```python
from build123d import *

# Parameters (mm, degrees)
SKETCH_1_W          = 160
SKETCH_1_H          = 25
EXTRUDE_1_DEPTH     = 4
SKETCH_3_R          = 1.45
CUT_EXTRUDE_1_DEPTH = 4
SKETCH_5_W          = 102
SKETCH_5_H          = 10
EXTRUDE_2_DEPTH     = 8
SKETCH_6_W          = 29
SKETCH_6_H          = 10
CUT_EXTRUDE_2_DEPTH = 6
CHAMFER_1_SIZE      = 10
CUT_EXTRUDE_3_DEPTH = 10
CUT_EXTRUDE_4_DEPTH = 142
SKETCH_10_W         = 122
SKETCH_10_H         = 12
CUT_EXTRUDE_5_DEPTH = 142
CHAMFER_2_SIZE      = 12
SKETCH_11_W         = 15
SKETCH_11_H         = 4
CUT_EXTRUDE_6_DEPTH = 1
SKETCH_12_W         = 15
SKETCH_12_H         = 4
CUT_EXTRUDE_7_DEPTH = 1


with BuildPart() as part:
    # 草图1 → 凸台-拉伸1 (new body)
    with BuildSketch(Plane(origin=(0, 0, 0), x_dir=(1, 0, 0), z_dir=(0, 1, 0))):
        Rectangle(SKETCH_1_W, SKETCH_1_H)
    extrude(amount=EXTRUDE_1_DEPTH)

    # 草图3 → 切除-拉伸1 (cut)
    with BuildSketch(Plane(origin=(0, 4, 0), x_dir=(1, 0, 0), z_dir=(0, 1, 0))):
        with Locations(Location((-75, 7.5, 0), (0, 0, 270))):
            Circle(SKETCH_3_R)
        with Locations(Location((75, 7.5, 0), (0, 0, 270))):
            Circle(SKETCH_3_R)
    extrude(amount=-CUT_EXTRUDE_1_DEPTH, mode=Mode.SUBTRACT)

    # 草图5 → 凸台-拉伸2 (add)
    with BuildSketch(Plane(origin=(0, 4, 0), x_dir=(1, 0, 0), z_dir=(0, 1, 0))):
        with Locations((0, -7.5)):
            Rectangle(SKETCH_5_W, SKETCH_5_H)
    extrude(amount=EXTRUDE_2_DEPTH)

    # 草图6 → 切除-拉伸2 (cut)
    with BuildSketch(Plane(origin=(0, 4, 0), x_dir=(1, 0, 0), z_dir=(0, 1, 0))):
        with Locations((-65.5, -7.5)):
            Rectangle(SKETCH_6_W, SKETCH_6_H)
        with Locations((65.5, -7.5)):
            Rectangle(SKETCH_6_W, SKETCH_6_H)
    extrude(amount=-CUT_EXTRUDE_2_DEPTH, mode=Mode.SUBTRACT)

    # 倒角1
    chamfer_1_edges = [part.edges().sort_by_distance(p)[0] for p in [
        (51, 2, 2.5),
        (-51, 2, 2.5),
    ]]
    chamfer(chamfer_1_edges, length=CHAMFER_1_SIZE - 0.0001)  # a hair under: the kernel refuses the full size

    # 草图7 → 切除-拉伸3 (cut)
    with BuildSketch(Plane(origin=(0, 12, 0), x_dir=(1, 0, 0), z_dir=(0, 1, 0))):
        Polygon((-39.8, -9.3), (-27.4, -9.3), (-27.4, -10.5), (-29.4, -10.5), (-29.4, -12.5), (-37.8, -12.5), (-37.8, -10.5), (-39.8, -10.5), align=None)
        Polygon((-17.4, -9.3), (-5, -9.3), (-5, -10.5), (-7, -10.5), (-7, -12.5), (-15.4, -12.5), (-15.4, -10.5), (-17.4, -10.5), align=None)
        Polygon((5, -9.3), (17.4, -9.3), (17.4, -10.5), (15.4, -10.5), (15.4, -12.5), (7, -12.5), (7, -10.5), (5, -10.5), align=None)
        Polygon((27.4, -9.3), (39.8, -9.3), (39.8, -10.5), (37.8, -10.5), (37.8, -12.5), (29.4, -12.5), (29.4, -10.5), (27.4, -10.5), align=None)
    extrude(amount=-CUT_EXTRUDE_3_DEPTH, mode=Mode.SUBTRACT)

    # 草图9 → 切除-拉伸4 (cut)
    with BuildSketch(Plane.ZY.offset(51)):
        Polygon((7.5, 12), (2.5, 4), (2.5, 12), align=None)
    extrude(amount=-CUT_EXTRUDE_4_DEPTH, mode=Mode.SUBTRACT)

    # 草图10 → 切除-拉伸5 (cut)
    with BuildSketch(Plane(origin=(0, 4, 0), x_dir=(1, 0, 0), z_dir=(0, 1, 0))):
        with Locations((0, 6.5)):
            Rectangle(SKETCH_10_W, SKETCH_10_H)
    extrude(amount=-CUT_EXTRUDE_5_DEPTH, mode=Mode.SUBTRACT)

    # 倒角2
    chamfer_2_edges = [part.edges().sort_by_distance(p)[0] for p in [
        (-61, 2, -0.5),
        (61, 2, -0.5),
    ]]
    chamfer(chamfer_2_edges, length=CHAMFER_2_SIZE - 0.0001)  # a hair under: the kernel refuses the full size

    # 草图11 → 切除-拉伸6 (cut)
    with BuildSketch(Plane.ZY.offset(80)):
        with Locations((-5, 2)):
            Rectangle(SKETCH_11_W, SKETCH_11_H)
    extrude(amount=-CUT_EXTRUDE_6_DEPTH, mode=Mode.SUBTRACT)

    # 草图12 → 切除-拉伸7 (cut)
    with BuildSketch(Plane(origin=(80, 0, 0), x_dir=(0, 0, -1), z_dir=(1, 0, 0))):
        with Locations((5, 2)):
            Rectangle(SKETCH_12_W, SKETCH_12_H)
    extrude(amount=-CUT_EXTRUDE_7_DEPTH, mode=Mode.SUBTRACT)


solid = part.part
```
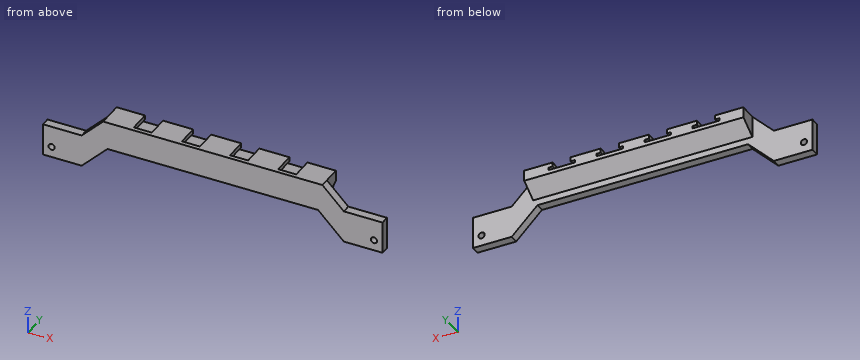
Geometry check sheet. Reference: the model listing, model coordinates, mm. Coordinates: 2 decimals unless noted, no trailing zeros. Write each loop counter-clockwise with the first axis right and the second up, starting at its lowest first coordinate (ties: lowest second). Pieces come first, ordered by that corner, then holes. Notation, with made-up numbers: M 56.5,-5.5 L 99.5,-5.5 A12 ccw 99.5,14.5 Z; hole C 86.5,0 d7. An arc over 180 degrees is marked long. Answer as a JSON object with one key per item and string values.
1. Scan lines: L1, parallel to Z at x = 75, y = 1.8; L2, parallel to X at y = 2.5, z = -7.5; L3, parallel to X at y = 9.5, z = 11. Record each from-to range of solid material in increasing order.
Answers below:
{"L1": "z = -12.5 to -8.95, -6.05 to 2.5", "L2": "x = -79 to -76.45, -73.55 to -56, 56 to 73.55, 76.45 to 79", "L3": "x = -51 to -37.8, -29.4 to -15.4, -7 to 7, 15.4 to 29.4, 37.8 to 51"}
2. Section check A-A, the plane x = -75. Enter the section's corners in (y, z), plus the area to 3 significant figures.
Answers below:
{"outline": "M 0,-12.5 L 4,-12.5 L 4,-8.95 L 0,-8.95 Z; M 0,-6.05 L 4,-6.05 L 4,2.5 L 0,2.5 Z", "area": "48.4 mm²"}
3. Section check C-C, the plane x = 54. Enter the section's corners in (y, z), plus the area to 3 significant figures.
Answers below:
{"outline": "M 0,-5.5 L 4,-5.5 L 4,9.5 L 0,9.5 Z", "area": "60.0 mm²"}
4. Section check B-B, the plane z = -7.5. Enter the section's corners in (x, y).
Answers below:
{"outline": "M -79,0 L -76.45,0 L -76.45,4 L -79,4 Z; M -73.55,0 L -56,0 L -56,4 L -73.55,4 Z; M 56,0 L 73.55,0 L 73.55,4 L 56,4 Z; M 76.45,0 L 79,0 L 79,4 L 76.45,4 Z"}
5. Go/stop test with flat-tipped pins: pin 1 Ø2 at (x, y) = (66.5, 2.5) entering from +Z; pin 2 Ø2 at (x, z) = (-50, 5.5) entering from +Y; pin 3 Ø1 at (x, y) = (-38.5, 1.5) entering from -Z. Record where each tip stops, or that it passes through.
Answers below:
{"pin 1": "stops at z = 2.5", "pin 2": "stops at y = 10.4", "pin 3": "stops at z = -0.5"}
